The model under review builds one solid part; all positions refer to its coordinate system, in mm. A direction names the side the tool comes from. Give positions to 0.01 mm unless a question says otherwise; leave off trailing zeros. Loops run counter-clockwise (first coordinate to the right, second up) from the corner with the lowest first, then second, coordinate; pieces in that order, holes last. Notation, with made-up numbers: M 11.5,-17.75 L 68.5,-17.75 A34 cw 68.5,14.25 Z; hole C 86,-29.75 d9. An arc over 180 degrees is marked long. Put each result on its own line as item: value. Start each with the question number.
```python
from build123d import *

# Parameters (mm, degrees)
F1_DEPTH = 54.102
F2_D     = 9.525
F3_W     = 74.6125
F3_H     = 28.702
F3_W_2   = 36.2260771513
F4_W     = 161.925
F4_H     = 27.051
F5_DEPTH = 25.4
F7_R     = 6.604


# Not quite as in the source:
# - a pattern or mirror of a feature is missing from the dataset's text; its kind, count and spacing are read off the source's solid


with BuildPart() as f1:
    # F0 (on Top) → F1 (new body)
    with BuildSketch(Plane.XY):
        with BuildLine():
            ThreePointArc((236.5375, -7.9375), (234.2126600757, -2.3248399243), (228.6, 0))
            Line((228.6, 0), (228.6, -15.875))
            ThreePointArc((228.6, -15.875), (234.2126600757, -13.5501600757), (236.5375, -7.9375))
        make_face()
        with BuildLine():
            Line((228.6, -15.875), (228.6, 0))
            ThreePointArc((228.6, 0), (220.6625, -7.9375), (228.6, -15.875))
        make_face()
        with BuildLine():
            Line((228.6, 0), (0, 0))
            ThreePointArc((0, 0), (5.6126600757, -2.3248399243), (7.9375, -7.9375))
            ThreePointArc((7.9375, -7.9375), (5.6126600757, -13.5501600757), (0, -15.875))
            Line((0, -15.875), (228.6, -15.875))
            ThreePointArc((228.6, -15.875), (220.6625, -7.9375), (228.6, 0))
        make_face()
        with BuildLine():
            ThreePointArc((7.9375, -7.9375), (5.6126600757, -2.3248399243), (0, 0))
            Line((0, 0), (0, -15.875))
            ThreePointArc((0, -15.875), (5.6126600757, -13.5501600757), (7.9375, -7.9375))
        make_face()
        with BuildLine():
            Line((0, -15.875), (0, 0))
            ThreePointArc((0, 0), (-7.9375, -7.9375), (0, -15.875))
        make_face()
    extrude(amount=F1_DEPTH)

    # F2 (through all)
    with Locations(Plane(origin=(0, 0, 0), x_dir=(1, 0, 0), z_dir=(0, 0, -1))):
        with Locations((0, 7.9375), (177.8, 7.9375), (228.6, 7.9375)):
            Hole(F2_D / 2)

    # F3 (on Front) + F4 (on Front) → F5 (cut)
    with BuildSketch(Plane.XZ):
        with Locations((191.29375, 27.051)):
            Rectangle(F3_W, F3_H)
        with Locations((246.7130385756, 27.051)):
            Rectangle(F3_W_2, F3_H)
    with BuildSketch(Plane.XZ):
        with Locations((60.325, 53.2765)):
            Rectangle(F4_W, F4_H)
    f5 = extrude(amount=F5_DEPTH, mode=Mode.SUBTRACT)

    # F5_copies: F5 across plane
    add(f5.mirror(Plane(origin=(0, 0, 27.051), x_dir=(-1, 0, 0), z_dir=(0, 0, -1))), mode=Mode.SUBTRACT)

    # F7
    f7_edges = [f1.edges().sort_by_distance(p)[0] for p in [
        (141.2875, -7.9375, 39.751),
        (141.2875, -7.9375, 54.102),
        (153.9875, -7.9375, 12.7),
        (153.9875, -7.9375, 41.402),
        (141.2875, -7.9375, 0),
        (141.2875, -7.9375, 14.351),
    ]]
    fillet(f7_edges, radius=F7_R)


solid = f1.part
```
Item 1: Clearance check with flat-ended pins moving along their axes: pin 1 Ø5 at (x, y) = (188.5, -6.5) entering from -Z; pin 2 Ø8.5 at (x, y) = (228.6, -7.94) entering from -Z; pin 3 Ø6 at (x, y) = (28, -13) entering from +Z; pin 4 Ø1 at (y, z) = (-13, 35) entering from +X. State where each tip first meets the part, or that it passes through.
Item 2: Draft analysis for pull direction X (two halves, no side actions). For faces 1 (the flat face through (192, -8, 54.102)), 2 (the cylindrical face through (173.4, -6.11, 47.84)), 3 (the cylindrical face through (143.171, -8.049, 52.116)), state which applies: +X half, -X half, draft (parallel to the pull), parting line (faces both ways), or undercut.
Item 3: Consider section A-A, the plane x = 177.8. Write out the cut boundary in (y, z) (3 decimals), plus the area to 3 significant figures.
Item 4: Tool access review of faces 4 (the cylindrical face through (155.973, -8.049, 14.583)), 5 (the flat face through (62, -8, 39.751)), 6 (the cylindrical face through (224.06, -9.37, 47.84)), 7 (the flat face through (62, -8, 14.351)), 8 (the flat face through (116, 0, 27)): name each direction out of +Z, -Z, +X, -X, +Y, -Y from which nothing blocks a thin tool from reaching the whole face with its end or side.
Item 5: Consider section D-D, the plane x = 33. Write out the cut boundary in (y, z) (3 decimals), plus the area to 3 significant figures.
Item 6: To check wall thickness, follow L1, parallel to Y at x = 228, z = 44 (3 decimals); L2, parallel to Z at x = 182.5, y = -2.25; L3, parallel to Z at x = 101, y = -1.5. State the ranges of each line that lie inside material, in increasing order. Write a range as [from, to].
Item 7: Consider section B-B, the plane x = 209. Write out the cut boundary in (y, z) (3 decimals).
Item 8: Consider section C-C, the plane z = 37.5. Write out the cut boundary in (x, y) (1 decimal), plus the area to 3 significant figures.
Report:
1. pin 1: z = 0
1. pin 2: through
1. pin 3: z = 39.75
1. pin 4: x = 154.02
2. face 1: draft
2. face 2: undercut
2. face 3: -X half
3. outline: M -15.875,0 L -12.7,0 L -12.7,12.7 L -15.875,12.7 Z; M -15.875,41.402 L -12.7,41.402 L -12.7,54.102 L -15.875,54.102 Z; M -3.175,0 L 0,0 L 0,12.7 L -3.175,12.7 Z; M -3.175,41.402 L 0,41.402 L 0,54.102 L -3.175,54.102 Z
3. area: 161 mm²
4. face 4: +X, +Y, -Y
4. face 5: +Z, -X, +Y, -Y
4. face 6: +Z, -Z
4. face 7: -Z, -X, +Y, -Y
4. face 8: +Z, -Z, +X, -X, +Y
5. outline: M -15.875,14.351 L 0,14.351 L 0,39.751 L -15.875,39.751 Z
5. area: 403 mm²
6. L1: [-15.875, -12.662], [-3.213, 0]
6. L2: [0, 12.7], [41.4, 54.1]
6. L3: [14.35, 39.75]
7. outline: M -15.875,0 L 0,0 L 0,12.7 L -15.875,12.7 Z; M -15.875,41.402 L 0,41.402 L 0,54.102 L -15.875,54.102 Z
8. outline: M 0,-15.9 L 154.6,-15.9 L 154.6,0 L 0,0 A7.9 ccw Z; hole C 0,-7.9 d9.5
8. area: 2,480 mm²
